Source: CAD feature listing. Evaluate the final solid. Frame: model axes, mm. Face numbers are marked on the shaded views. A direction names the side the tool comes from. Give positions to 0.01 mm unless a question says otherwise; leave off trailing zeros. Loops run counter-clockwise (first coordinate to the right, second up) from the corner with the lowest first, then second, coordinate; pieces in that order, holes last.
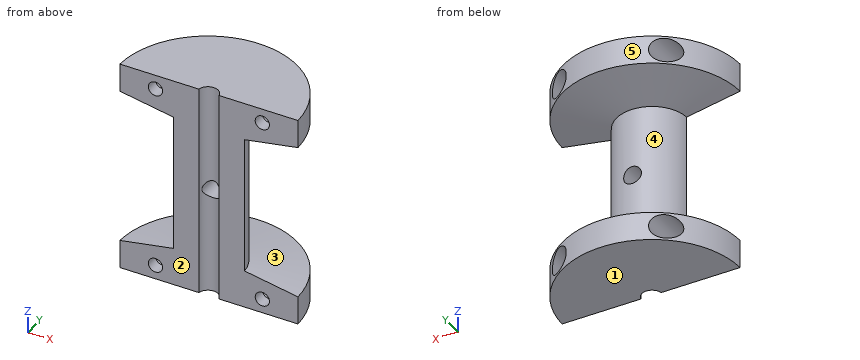
Autodesk Inventor part; units mm, degrees
ref_plane "Plan de construction2" through (0, 25, -60) normal (0, 1, 0) x (-1, 0, 0)
ref_plane "YZ Plane" through (0, 0, 0) normal (1, 0, 0) x (0, 1, 0)
ref_plane "XZ Plane" through (0, 0, 0) normal (0, 1, 0) x (-1, 0, 0)
sketch "Esquisse1" plane through (0, 0, 0) normal (1, 0, 0) x (0, 1, 0)
  line L0 (0, 0) -> (0, -46.4485)
  line L1 (2.875, 0) -> (25, 0)
  line L2 (25, 0) -> (25, -8)
  line L3 (2.875, 0) -> (2.875, -60)
  line L4 (25, -8) -> (10, -10.6449)
  line L5 (10, -10.6449) -> (10, -49.3551)
  line L6 (10, -49.3551) -> (25, -52)
  line L7 (25, -52) -> (25, -60)
  line L8 (2.875, -60) -> (25, -60)
  dimension "d0" = 5.75
  dimension "d1" = 50
  dimension "d2" = 20
  dimension "d3" = 100
  dimension "d4" = 8
  dimension "d5" = 100
  dimension "d6" = 60
  dimension "d7" = 15
  dimension "d8" = 38.7102
revolve "Révolution1" add sketch "Esquisse1" angle 360 about axis through (0, 0, 0) along (0, 0, -1)
sketch "Esquisse2" plane through (0, 0, 0) normal (0, 0, 1) x (1, 0, 0)
  circle A0 centre (0, 0) radius 25
  line L0 (-25, 0.5) -> (25, 0.5)
  line L1 (25, 0.5) -> (25, -25)
  line L2 (25, -25) -> (-25, -25)
  line L3 (-25, -25) -> (-25, 0.5)
  point P0 (-25, 0)
  point P1 (25, 0)
  dimension "d42" = 0.5
extrude "Extrusion1" cut sketch "Esquisse2" against normal up to surface (60 mm away) contours A0 L0 | L1 L2 A0 | A0 L0 L1 | L2 L3 A0 | A0 L3 L0 picked at (-6.5153, -4.8624)
sketch "Esquisse3" plane through (-25, 0.5, 0) normal (0, -1, 0) x (1, 0, 0)
  line L0 (0, -52) -> (15, -49.3551)
  line L1 (0, -60) -> (0, -52)
  line L2 (22.125, -60) -> (0, -60)
  line L3 (22.125, 0) -> (22.125, -60)
  line L4 (0, 0) -> (22.125, 0)
  line L5 (0, -8) -> (0, 0)
  line L6 (15, -10.6449) -> (0, -8)
  line L7 (15, -49.3551) -> (15, -10.6449)
  line L8 (35, -49.3551) -> (50, -52)
  line L9 (35, -10.6449) -> (35, -49.3551)
  line L10 (50, -8) -> (35, -10.6449)
  line L11 (50, 0) -> (50, -8)
  line L12 (27.875, 0) -> (50, 0)
  line L13 (27.875, -60) -> (27.875, 0)
  line L14 (50, -60) -> (27.875, -60)
  line L15 (50, -52) -> (50, -60)
  line L16 (22.1688, -60) -> (27.8312, -60)
  line L17 (22.1688, 0) -> (27.8312, 0)
  circle A0 centre (25, -30) radius 2.5
  line L18 (27.8312, -60) -> (27.8312, 0)
  line L19 (22.1688, 0) -> (22.1688, -60)
  point P0 (25, 0)
  point P1 (22.125, 0)
  point P2 (27.875, 0)
  point P3 (25, 0)
  dimension "d13" = 60
  dimension "d14" = 30
  dimension "d15" = 5
extrude "Extrusion2" cut sketch "Esquisse3" against normal up to surface contours A0
ref_plane "Plan de construction2" through (0, 25, -60) normal (0, 1, 0) x (-1, 0, 0)
sketch "Esquisse6" plane through (0, 25, -60) normal (0, 1, 0) x (-1, 0, 0)
  line L0 (24.995, 0) -> (-24.995, 0)
  line L1 (24.995, 8) -> (-24.995, 8)
  line L2 (24.995, 52) -> (-24.995, 52)
  line L3 (24.995, 60) -> (-24.995, 60)
  line L4 (-24.995, 60) -> (-24.995, 52)
  line L5 (24.995, 52) -> (24.995, 60)
  line L6 (-24.995, 8) -> (-24.995, 0)
  line L7 (24.995, 0) -> (24.995, 8)
  point P0 (0, 60)
  point P1 (25, 8)
  point P2 (25, 0)
  point P3 (-25, 0)
  point P4 (-25, 8)
  point P5 (25, 60)
  point P6 (25, 52)
  point P7 (-25, 52)
  point P8 (-25, 60)
  point P9 (-15, 4)
  point P10 (15, 4)
  point P11 (15, 56)
  point P12 (-15, 56)
  dimension "d31" = 8
  dimension "d32" = 4
  dimension "d33" = 4
hole "Perçage2" at (15, 25, -56) at (-15, 25, -56) at (-15, 25, -4) at (15, 25, -4) direction (0, -1, 0) diameter 4 end through all counterbore diameter 6.9 counterbore depth 21
equation "\"d5\" = d3"
equation "\"d14\" = 0.5 * d13"
properties part number "demi_tambour"
(1) Section D-D, the plane y = 16. Count the separate pieces of the cut face and the enclosed holes in it, then the cut area to 3 significant figures.
A:
separate pieces: 2
enclosed holes: 4
area: 543 mm2
(2) Section C-C, the plane z = -56. Return the cut outline in (x, y) (3 decimals), then the cut area to 3 significant figures.
A:
outline: (-24.995, 0.5) - (-17, 0.5) - (-17, 4) - (-18.45, 4) - (-18.45, 16.87) arc R25 ccw to start; (-13, 0.5) - (-2.831, 0.5) arc R2.875 cw to (2.831, 0.5) - (13, 0.5) - (13, 4) - (11.55, 4) - (11.55, 22.172) arc R25 ccw to (-11.55, 22.172) - (-11.55, 4) - (-13, 4) - close; (17, 0.5) - (24.995, 0.5) arc R25 ccw to (18.45, 16.87) - (18.45, 4) - (17, 4) - close
area: 700 mm2
(3) Reachability of the marked faces 4 and 5 from +Z, -Z, +X, -X, +Y, -Y: full face, straight path, thin tool, end or side. Return the list, or none.
A:
face 4: +Y
face 5: +Z, -Z, +Y
(4) Mould query, pull axis Z, two halves, no side actions, for the marked faces 1, 2 and 3. Classes: pulls with the +Z half, pulls with the -Z half, needs draft (parallel to the pull), parting line crosses it, or undercut.
A:
face 1: pulls with the -Z half
face 2: needs draft
face 3: undercut
(5) Section B-B, the plane x = 0. Return the cut outline in (y, z) (3 decimals), then the cut area to 3 significant figures.
A:
outline: (2.875, -60) - (25, -60) - (25, -52) - (10, -49.355) - (10, -32.5) - (2.875, -32.5) - close; (2.875, -27.5) - (10, -27.5) - (10, -10.645) - (25, -8) - (25, 0) - (2.875, 0) - close
area: 672 mm2
(6) First-contact query: pin 1 (6.5 mm diameter, centred on x = 15, z = -56, fed in from +Y); pin 2 (4 mm diameter, centred on x = 1.5, z = -11, fed in from -Y); pin 3 (2.5 mm diameter, centred on x = 15, z = -4, fed in from -Y); pin 4 (10 mm diameter, centred on x = 6, z = -20.5, fed in from +Y). Flat tips, straight axial feed; report the tip coordinate or a pass-through.
A:
pin 1: stops at y = 4
pin 2: stops at y = 0.5
pin 3: passes through
pin 4: stops at y = 9.95
(7) Ray query, line 1 along X through (y, z) = (12, -4); line 2 along X through (y, z) = (8.5, -4); line 3 along Z through (x, y) = (-15, 8.25). Return the intervals inside material, ascending.
A:
line 1: x = -21.93 to -18.45, -11.55 to 11.55, 18.45 to 21.93
line 2: x = -23.51 to -18.45, -11.55 to 11.55, 18.45 to 23.51
line 3: z = -60 to -59.45, -52.55 to -50.61, -9.39 to -7.45, -0.55 to 0
